Build history of the part. All positions in model axes, mm. Round coordinates to 2 decimals unless told otherwise and drop trailing zeros. Loops run counter-clockwise (first coordinate to the right, second up) from the corner with the lowest first, then second, coordinate; pieces in that order, holes last. Notation, with made-up numbers: M -6.75,9.5 L 43.25,9.5 A23 ccw 43.25,22.5 Z; hole C 36,79 d4. An arc over 180 degrees is marked long. Use one line per item in the form item = value. Start each with the question number.
```python
from build123d import *

# Parameters (mm, degrees)
SKETCH_1_R          = 2
SKETCH_1_R_2        = 1.5
EXTRUDE_1_DEPTH     = 3
SKETCH_2_W          = 20
SKETCH_2_H          = 3
CUT_EXTRUDE_1_DEPTH = 80.755877526
SKETCH_3_R          = 1
CUT_EXTRUDE_2_DEPTH = 80.755877526
FILLET_1_R          = 1
FILLET_2_R          = 3


with BuildPart() as part:
    # 草图1 → 凸台-拉伸1 (new body)
    with BuildSketch(Plane(origin=(0, 0, 0), x_dir=(1, 0, 0), z_dir=(0, 1, 0))):
        Polygon((-53.5, 24), (-53.5, 9), (-7.5, 9), (-7.5, 24), (7.5, 24), (7.5, 9), (53.5, 9), (53.5, 24), (76, 24), (76, 9), (67, 0), (-67, 0), (-76, 9), (-76, 24), align=None)
        with Locations(Location((-61, 16.5, 0), (0, 0, 270))):
            Circle(SKETCH_1_R, mode=Mode.SUBTRACT)
        with Locations(Location((-52.5, 3, 0), (0, 0, 270))):
            Circle(SKETCH_1_R_2, mode=Mode.SUBTRACT)
        with Locations(Location((-17.5, 3, 0), (0, 0, 270))):
            Circle(SKETCH_1_R_2, mode=Mode.SUBTRACT)
        with Locations(Location((0, 16.5, 0), (0, 0, 270))):
            Circle(SKETCH_1_R, mode=Mode.SUBTRACT)
        with Locations(Location((17.5, 3, 0), (0, 0, 90))):
            Circle(SKETCH_1_R_2, mode=Mode.SUBTRACT)
        with Locations(Location((52.5, 3, 0), (0, 0, 90))):
            Circle(SKETCH_1_R_2, mode=Mode.SUBTRACT)
        with Locations(Location((61, 16.5, 0), (0, 0, 90))):
            Circle(SKETCH_1_R, mode=Mode.SUBTRACT)
    extrude(amount=EXTRUDE_1_DEPTH)

    # 草图2 → 切除-拉伸1 (cut, through all)
    with BuildSketch(Plane(origin=(0, 3, 0), x_dir=(1, 0, 0), z_dir=(0, 1, 0))):
        with Locations((35, 7.5)):
            Rectangle(SKETCH_2_W, SKETCH_2_H)
        with Locations((-35, 7.5)):
            Rectangle(SKETCH_2_W, SKETCH_2_H)
        Polygon((-69.014718626, 10.5), (-59.5, 10.5), (-59.5, 6), (-64.514718626, 6), align=None)
        Polygon((64.514718626, 6), (59.5, 6), (59.5, 10.5), (69.014718626, 10.5), align=None)
    extrude(amount=-CUT_EXTRUDE_1_DEPTH, mode=Mode.SUBTRACT)

    # 草图3 → 切除-拉伸2 (cut, through all)
    with BuildSketch(Plane(origin=(0, 3, 0), x_dir=(1, 0, 0), z_dir=(0, 1, 0))):
        with Locations((-53.5, 10)):
            Circle(SKETCH_3_R)
        with Locations((-44, 6)):
            Circle(SKETCH_3_R)
        with Locations((-26, 6)):
            Circle(SKETCH_3_R)
        with Locations((26, 6)):
            Circle(SKETCH_3_R)
        with Locations((44, 6)):
            Circle(SKETCH_3_R)
        with Locations((53.5, 10)):
            Circle(SKETCH_3_R)
    extrude(amount=-CUT_EXTRUDE_2_DEPTH, mode=Mode.SUBTRACT)

    # 圆角1
    fillet_1_edges = [part.edges().sort_by_distance(p)[0] for p in [
        (45, 1.5, -9),
        (25, 1.5, -9),
        (-45, 1.5, -9),
        (-25, 1.5, -9),
        (-76, 1.5, -24),
        (-53.5, 1.5, -24),
        (-7.5, 1.5, -9),
        (-7.5, 1.5, -24),
        (7.5, 1.5, -24),
        (7.5, 1.5, -9),
        (53.5, 1.5, -24),
        (76, 1.5, -24),
        (69.014718626, 1.5, -10.5),
        (59.5, 1.5, -6),
        (59.5, 1.5, -10.5),
        (-59.5, 1.5, -6),
        (-69.014718626, 1.5, -10.5),
        (-59.5, 1.5, -10.5),
    ]]
    fillet(fillet_1_edges, radius=FILLET_1_R)

    # 圆角2
    fillet_2_edges = [part.edges().sort_by_distance(p)[0] for p in [
        (76, 1.5, -9),
        (67, 1.5, 0),
        (-67, 1.5, 0),
        (-76, 1.5, -9),
        (64.514718626, 1.5, -6),
        (-64.514718626, 1.5, -6),
    ]]
    fillet(fillet_2_edges, radius=FILLET_2_R)


solid = part.part
```
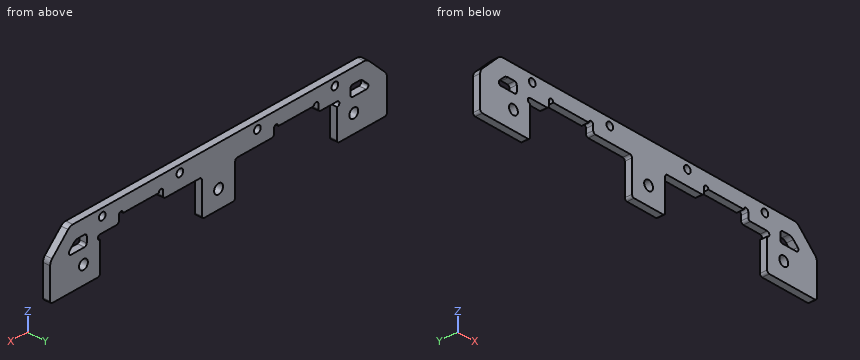
Q1. Saw through at B-B (z = -3). Give the cut face in (x, y).
Q2. Saw through at C-C (x = 14.5). Give the cut face in (y, z).
Q3. Wall check: probe 1 along X at (y, z) = (1.35, -22); probe 2 along Z at (x, y) = (61, 1.55); probe 3 along X at (y, z) = (2.1, -3). Give the ranges that are in metal, low to high.
Q4. Drop flat-ended pins along their axis: P1, Ø1.6, axis at y = 2, z = -7, coming from the -X side; P2, Ø1.6, axis at y = 1.5, z = -7, coming from the +X side; P3, Ø1.5, axis at x = -33.5, y = 1, coming from the -Z side. Give the stop position or say it passes through.
Q5. Saw through at D-D (y = 2.1). Give the number of separate pieces and of enclosed holes in the cut face, and give its area (3 significant figures).
Q6. Saw through at A-A (z = -12.75). Give the cut face in (x, y), and give its area (3 significant figures).
Filled in:
q1.outline = M -70,0 L -54,0 L -54,3 L -70,3 Z; M -51,0 L -19,0 L -19,3 L -51,3 Z; M -16,0 L 16,0 L 16,3 L -16,3 Z; M 19,0 L 51,0 L 51,3 L 19,3 Z; M 54,0 L 70,0 L 70,3 L 54,3 Z
q2.outline = M 0,-9 L 3,-9 L 3,0 L 0,0 Z
q3.probe_1 = -76 to -53.5, -7.5 to 7.5, 53.5 to 76
q3.probe_2 = -24 to -18.5, -14.5 to -10.5, -6 to 0
q3.probe_3 = -70 to -54, -51 to -19, -16 to 16, 19 to 51, 54 to 70
q4.P1 = -74.8
q4.P2 = 74.8
q4.P3 = -6
q5.separate_pieces = 1
q5.enclosed_holes = 9
q5.area = 1,930 mm²
q6.outline = M -76,0 L -53.5,0 L -53.5,3 L -76,3 Z; M -7.5,0 L 7.5,0 L 7.5,3 L -7.5,3 Z; M 53.5,0 L 76,0 L 76,3 L 53.5,3 Z
q6.area = 180 mm²
